Read the model definition and answer for the solid it produces. Units are mm, in the model's axes. A direction names the side the tool comes from. Give positions to 0.01 mm unless a question says otherwise; leave off trailing zeros. Write each loop counter-clockwise with the first axis right and the second up, starting at its lowest first coordinate (ties: lowest second). Pieces come first, ordered by that corner, then holes. Notation, with made-up numbers: M 49.25,-13.75 L 94.25,-13.75 A18 ccw 94.25,-4.75 Z; hole C -1.75,51 d8. An arc over 180 degrees is marked long. Write each question's results on one line, items separated by ' | '. Start each with the question number.
```python
from build123d import *

# Parameters (mm, degrees)
F6_DEPTH  = 8.89
F7_R      = 6.35
F8_DEPTH  = 25.4
F9_R      = 5.3975
F10_DEPTH = 4.318
F11_R     = 3.556
F12_DEPTH = 0.889
F13_R     = 2.3495
F14_DEPTH = 9.7282


# Not quite as in the source:
# - a variable given as a bare number and used for a length is read in inches; the dataset says mm whatever the document's units were


with BuildPart() as f6:
    # F5 (on Top) → F6 (new body)
    with BuildSketch(Plane.XY):
        Polygon((5.499261314, 9.525), (-5.499261314, 9.525), (-10.9985226281, 0), (-5.499261314, -9.525), (5.499261314, -9.525), (10.9985226281, 0), align=None)
    extrude(amount=F6_DEPTH)

    # F7 (on face) → F8 (join)
    with BuildSketch(Plane.XY.offset(8.89)):
        Circle(F7_R)
    extrude(amount=F8_DEPTH)

    # F9 (on face) → F10 (join)
    with BuildSketch(Plane.XY.offset(34.29)):
        Circle(F9_R)
    extrude(amount=F10_DEPTH)

    # F11 (on face) → F12 (cut)
    with BuildSketch(Plane.XY.offset(38.608)):
        Circle(F11_R)
    extrude(amount=-F12_DEPTH, mode=Mode.SUBTRACT)

    # F13 (on face) → F14 (cut)
    with BuildSketch(Plane.XY.offset(38.608)):
        Circle(F13_R)
    extrude(amount=-F14_DEPTH, mode=Mode.SUBTRACT)


solid = f6.part
```
Item 1: Determine the mould class of faces 1 (the flat face through (-8.287, -4.696, 4.383)), 2 (the flat face through (0, 0, 28.88)), 3 (the flat face through (8.287, 4.696, 4.383)), 4 (the cylindrical face through (-0.77, -3.47, 38.17)) for opening direction X: +X half, -X half, draft (parallel to the pull), parting line (faces both ways), or undercut.
Item 2: For faces 5 (the cylindrical face through (-3.978, 3.648, 36.419)), 6 (the flat face through (0, -9.525, 4)), determine the directions among +Z, -Z, +X, -X, +Y, -Y from which every point of the face is accessible in a straight line to the end or side of a thin tool.
Item 3: Section B-B, the plane z = 27.5 is taken. Determine the outline of the cut face in (x, y).
Item 4: Straight lines are drawn through the part: line 1 (Y direction, x = 0, z = 34.25); line 2 (Y direction, x = 0, z = 38); line 3 (Z direction, x = 6, y = -4.25). For each, find the intervals that lie inside material, in ascending order.
Item 5: Given P1, Ø1, axis at x = 4.5, z = 18, coming from the -Y side; P2, Ø1, axis at y = -1.5, z = 11, coming from the -X side; P3, Ø10, axis at y = 4.5, z = 28, coming from the +X side; P4, Ø2, axis at x = -8, z = 27, coming from the +Y side, each flat-ended and moving along its own axis, determine where each tip first touches the part or whether it passes through.
Item 6: Section D-D, the plane x = 4.25 is taken. Determine the outline of the cut face in (y, z) (3 decimals).
Item 7: Section C-C, the plane y = 1 is taken. Determine the outline of the cut face in (x, z), then the cut area to 3 significant figures.
Worked out:
1) face 1: -X half | face 2: undercut | face 3: +X half | face 4: undercut
2) face 5: +Z | face 6: +Z, -Z, +X, -X, -Y
3) outline: C 0,0 d12.7
4) line 1: y = -6.35 to -2.35, 2.35 to 6.35 | line 2: y = -5.4 to -3.56, 3.56 to 5.4 | line 3: z = 0 to 8.89
5) P1: stops at y = -4.93 | P2: stops at x = -6.27 | P3: stops at x = 6.35 | P4: passes through
6) outline: M -9.525,0 L 9.525,0 L 9.525,8.89 L 4.718,8.89 L 4.718,34.29 L 3.327,34.29 L 3.327,38.608 L -3.327,38.608 L -3.327,34.29 L -4.718,34.29 L -4.718,8.89 L -9.525,8.89 Z
7) outline: M -10.42,0 L 10.42,0 L 10.42,8.89 L 6.27,8.89 L 6.27,34.29 L 5.3,34.29 L 5.3,38.61 L 3.41,38.61 L 3.41,37.72 L 2.13,37.72 L 2.13,28.88 L -2.13,28.88 L -2.13,37.72 L -3.41,37.72 L -3.41,38.61 L -5.3,38.61 L -5.3,34.29 L -6.27,34.29 L -6.27,8.89 L -10.42,8.89 Z | area: 506 mm²
